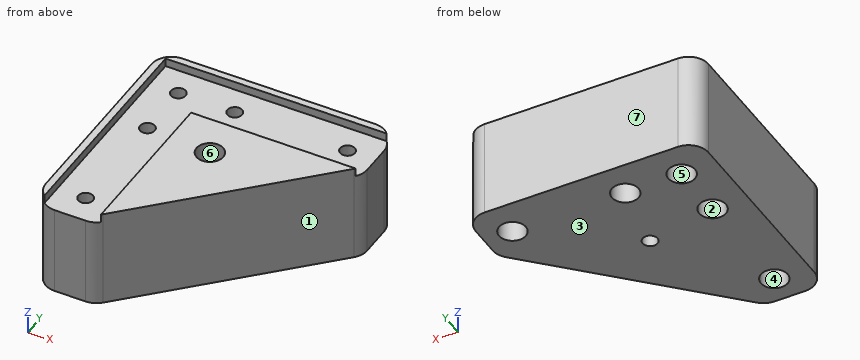
from build123d import *

# Parameters (mm, degrees)
SKETCH013_R          = 2.62
SKETCH013_R_2        = 2.65
PAD006_DEPTH         = 32
PAD006_DEPTH_BACK    = 3
SKETCH014_R          = 4.75
POCKET004_DEPTH      = 17
POCKET005_DEPTH      = 3.001
SKETCH109_R          = 4.75
POCKET055_DEPTH      = 22
POCKET055_DEPTH_BACK = 100


with BuildPart() as foot004:
    # Sketch013 → Pad006 (new body, two sides)
    with BuildSketch(Plane.XY) as pad006_sk:
        with BuildLine():
            Line((70, -5.5), (70, 5.5))
            ThreePointArc((70, 5.5), (69.467157, 8.178784), (67.949747, 10.449747))
            Line((67.949747, 10.449747), (10.449747, 67.949747))
            ThreePointArc((10.449747, 67.949747), (8.178784, 69.467157), (5.5, 70))
            Line((5.5, 70), (-5.5, 70))
            ThreePointArc((-5.5, 70), (-10.449747, 67.949747), (-12.5, 63))
            Line((-12.5, -5.5), (-12.5, 63))
            ThreePointArc((-12.5, -5.5), (-10.449747, -10.449747), (-5.5, -12.5))
            Line((-5.5, -12.5), (63, -12.5))
            ThreePointArc((63, -12.5), (67.949747, -10.449747), (70, -5.5))
        make_face()
        with Locations((20, 0)):
            Circle(SKETCH013_R, mode=Mode.SUBTRACT)
        with Locations((60, 0)):
            Circle(SKETCH013_R, mode=Mode.SUBTRACT)
        Circle(SKETCH013_R, mode=Mode.SUBTRACT)
        with Locations((0, 60)):
            Circle(SKETCH013_R, mode=Mode.SUBTRACT)
        with Locations((0, 20)):
            Circle(SKETCH013_R, mode=Mode.SUBTRACT)
        with Locations((24.748737, 24.748737)):
            Circle(SKETCH013_R_2, mode=Mode.SUBTRACT)
    extrude(amount=-PAD006_DEPTH)
    extrude(pad006_sk.sketch, amount=PAD006_DEPTH_BACK)

    # Sketch014 → Pocket004 (cut)
    with BuildSketch(Plane.XY.offset(-32)):
        with Locations((0, 60)):
            Circle(SKETCH014_R)
        Circle(SKETCH014_R)
        with Locations((20, 0)):
            Circle(SKETCH014_R)
        with Locations((60, 0)):
            Circle(SKETCH014_R)
        with Locations((0, 20)):
            Circle(SKETCH014_R)
    extrude(amount=POCKET004_DEPTH, mode=Mode.SUBTRACT)

    # Sketch016 → Pocket005 (cut, through all)
    with BuildSketch(Plane.XY):
        Polygon((10, 100), (10, 10), (140, 10), (140, -10), (-10, -10), (-10, 100), align=None)
    extrude(amount=POCKET005_DEPTH, mode=Mode.SUBTRACT)

    # Sketch109 → Pocket055 (cut, two sides)
    with BuildSketch(Plane.XY) as pocket055_sk:
        with Locations((24.748737, 24.748737)):
            Circle(SKETCH109_R)
    extrude(amount=-POCKET055_DEPTH, mode=Mode.SUBTRACT)
    extrude(pocket055_sk.sketch, amount=POCKET055_DEPTH_BACK, mode=Mode.SUBTRACT)


with BuildPart() as foot1:
    # Part__Mirroring: instance of Foot004
    add(foot004.part.mirror(Plane(origin=(38.75, -2e-06, -14.5), x_dir=(1, 0, 0), z_dir=(0, 1, 0))))


with BuildPart() as foot1_1:
    # Part__Mirroring placement: moved
    add(foot1.part.moved(Location((10, 686, 0))))


solid = foot1_1.part
The listing builds one solid part. Answer for the finished solid, in the listing's coordinates (mm). Face numbers are marked on the shaded views. A direction names the side the tool comes from. Give positions to 0.01 mm unless a question says otherwise; leave off trailing zeros. Write each loop counter-clockwise with the first axis right and the second up, starting at its lowest first coordinate (ties: lowest second). Pieces come first, ordered by that corner, then holes.
Item 1: Find the intervals of material crossed by line 1 along Y through (x, z) = (10, -4.75); line 2 along X through (y, z) = (683, -22.5); line 3 along Z through (x, y) = (13.5, 624.5), in increasing order.
Item 2: Which of the six approach directions +Z, -Z, +X, -X, +Y, -Y give full straight-line access (tool end or side, diameter ignored) to the marked faces 5, 6 and 7?
Item 3: Section B-B, the plane y = 636.5 is taken. Write down the section's boundary in (x, z).
Item 4: Section C-C, the plane z = -13.5 is taken. Write down the section's boundary in (x, y), plus the area to 3 significant figures.
Item 5: Section D-D, the plane x = 70 is taken. Write down the section's boundary in (y, z).
Item 6: Section A-A, the plane x = 10 is taken. Count the separate pieces of the cut face and the enclosed holes in it, plus the area to 3 significant figures.
Item 7: Flat-ended cylindrical pins translate along their axes: P1, Ø2, axis at y = 645, z = -1.5, coming from the +X side; P2, Ø4, axis at y = 675, z = -27, coming from the +X side; P3, Ø2.5, axis at x = 35.5, z = 1, coming from the -Y side. Find the tip coordinate at first contact, or state that the pin passes through.
Item 8: Determine the mould class of the marked faces 1, 2, 3 and 4 for opening direction X: released by +X, released by -X, zero draft, split by the parting line, or undercut.
Completed:
1. line 1: y = 616 to 623.38, 628.62 to 663.38, 668.62 to 683.38, 688.62 to 698.5
1. line 2: x = -2.5 to 6.32, 13.68 to 26.32, 33.68 to 66.32, 73.68 to 80
1. line 3: z = -15 to 0
2. face 5: -Z
2. face 6: +Z
2. face 7: +Z, -Z, +X, -X, +Y
3. outline: (-2.5, -32) - (38.9, -32) - (38.9, 3) - (20, 3) - (20, 0) - (0, 0) - (0, 3) - (-2.5, 3) - close
4. outline: (-2.5, 623) arc R7 ccw to (4.5, 616) - (15.5, 616) arc R7 ccw to (20.45, 618.05) - (77.95, 675.55) arc R7 ccw to (80, 680.5) - (80, 691.5) arc R7 ccw to (73, 698.5) - (4.5, 698.5) arc R7 ccw to (-2.5, 691.5) - close; hole circle Ø5.24 at (10, 626); hole circle Ø5.24 at (10, 666); hole circle Ø5.24 at (10, 686); hole circle Ø5.24 at (30, 686); hole circle Ø9.5 at (34.75, 661.25); hole circle Ø5.24 at (70, 686)
4. area: 4,700 mm2
5. outline: (667.6, -32) - (681.25, -32) - (681.25, -15) - (683.38, -15) - (683.38, 0) - (676, 0) - (676, 3) - (667.6, 3) - close; (688.62, -15) - (690.75, -15) - (690.75, -32) - (698.5, -32) - (698.5, 3) - (696, 3) - (696, 0) - (688.62, 0) - close
6. separate pieces: 4
6. enclosed holes: 0
6. area: 1,930 mm2
7. P1: stops at x = 48.4
7. P2: stops at x = 79.06
7. P3: stops at y = 631.85
8. face 1: released by +X
8. face 2: undercut
8. face 3: zero draft
8. face 4: undercut
